Design review of the part built by this model. Coordinates are the model's own, in mm. Give positions to 0.01 mm unless a question says otherwise; leave off trailing zeros. Order: outer loops, then holes, each group sorted by start corner. A loop starts at its lowest first (then second) coordinate and runs counter-clockwise, first axis right, second up. Notation, with made-up numbers: M 0,62 L 42,62 A14 cw 42,79 Z; hole C 83,52.5 d7. An arc over 180 degrees is marked long. Put each result on its own line as item: value. Start each with the question number.
from build123d import *

# Parameters (mm, degrees)
BOSS_EXTRUDE1_DEPTH = 3.175
SKETCH4_R           = 2.1
SKETCH4_R_2         = 2.249999999
SKETCH4_R_3         = 2.25
CUT_EXTRUDE2_DEPTH  = 343.045224939


with BuildPart() as part:
    # Sketch2 → Boss-Extrude1 (new body)
    with BuildSketch(Plane.XY):
        with BuildLine():
            Line((-166.376823509, -157.21600002), (-166.376823509, -168.26500002))
            Line((-166.376823509, -168.26500002), (-167.519823509, -168.26500002))
            Line((-167.519823509, -168.26500002), (-167.519823509, -174.61500002))
            Line((-167.519823509, -174.61500002), (-163.058823509, -174.61500002))
            Line((-163.058823509, -174.61500002), (-163.058823509, -187.31500002))
            Line((-163.058823509, -187.31500002), (-167.519823509, -187.31500002))
            Line((-167.519823509, -187.31500002), (-167.519823509, -193.66500002))
            Line((-167.519823509, -193.66500002), (-166.376823509, -193.66500002))
            Line((-166.376823509, -193.66500002), (-166.376823509, -194.18100002))
            Line((-166.376823509, -194.18100002), (-148.199823509, -194.18100002))
            Line((-148.199823509, -194.18100002), (-148.199823509, -203.71400002))
            Line((-148.199823509, -203.71400002), (255.426176451, -203.71400002))
            Line((255.426176451, -203.71400002), (255.426176451, -194.18100002))
            Line((255.426176451, -194.18100002), (273.603176451, -194.18100002))
            Line((273.603176451, -194.18100002), (273.603176451, -193.66500002))
            Line((273.603176451, -193.66500002), (274.746176451, -193.66500002))
            Line((274.746176451, -193.66500002), (274.746176451, -187.31500002))
            Line((274.746176451, -187.31500002), (270.285176451, -187.31500002))
            Line((270.285176451, -187.31500002), (270.285176451, -174.61500002))
            Line((270.285176451, -174.61500002), (274.746176451, -174.61500002))
            Line((274.746176451, -174.61500002), (274.746176451, -168.26500002))
            Line((274.746176451, -168.26500002), (273.603176451, -168.26500002))
            Line((273.603176451, -168.26500002), (273.603176451, -157.21600002))
            Line((273.603176451, -157.21600002), (255.463301471, -157.21600002))
            Line((255.463301471, -157.21600002), (255.463301471, -160.70800002))
            ThreePointArc((255.463301471, -160.70800002), (254.533365501, -162.95306405), (252.288301471, -163.88300002))
            Line((252.288301471, -163.88300002), (242.288301471, -163.88300002))
            ThreePointArc((242.288301471, -163.88300002), (240.04323744, -162.95306405), (239.113301471, -160.70800002))
            Line((239.113301471, -160.70800002), (239.113301471, -157.21600002))
            Line((239.113301471, -157.21600002), (220.538301471, -157.21600002))
            Line((220.538301471, -157.21600002), (220.538301471, -160.70800002))
            ThreePointArc((220.538301471, -160.70800002), (219.608365501, -162.95306405), (217.363301471, -163.88300002))
            Line((217.363301471, -163.88300002), (207.363301471, -163.88300002))
            ThreePointArc((207.363301471, -163.88300002), (205.11823744, -162.95306405), (204.188301471, -160.70800002))
            Line((204.188301471, -160.70800002), (204.188301471, -157.21600002))
            Line((204.188301471, -157.21600002), (175.452051471, -157.21600002))
            Line((175.452051471, -157.21600002), (175.452051471, -160.70800002))
            ThreePointArc((175.452051471, -160.70800002), (174.522115501, -162.95306405), (172.277051471, -163.88300002))
            Line((172.277051471, -163.88300002), (162.277051471, -163.88300002))
            ThreePointArc((162.277051471, -163.88300002), (160.03198744, -162.95306405), (159.102051471, -160.70800002))
            Line((159.102051471, -160.70800002), (159.102051471, -157.21600002))
            Line((159.102051471, -157.21600002), (140.527051471, -157.21600002))
            Line((140.527051471, -157.21600002), (140.527051471, -160.70800002))
            ThreePointArc((140.527051471, -160.70800002), (139.597115501, -162.95306405), (137.352051471, -163.88300002))
            Line((137.352051471, -163.88300002), (127.352051471, -163.88300002))
            ThreePointArc((127.352051471, -163.88300002), (125.10698744, -162.95306405), (124.177051471, -160.70800002))
            Line((124.177051471, -160.70800002), (124.177051471, -157.21600002))
            Line((124.177051471, -157.21600002), (73.849301471, -157.21600002))
            Line((73.849301471, -157.21600002), (73.849301471, -160.70800002))
            ThreePointArc((73.849301471, -160.70800002), (72.919365501, -162.95306405), (70.674301471, -163.88300002))
            Line((70.674301471, -163.88300002), (60.674301471, -163.88300002))
            ThreePointArc((60.674301471, -163.88300002), (58.42923744, -162.95306405), (57.499301471, -160.70800002))
            Line((57.499301471, -160.70800002), (57.499301471, -157.21600002))
            Line((57.499301471, -157.21600002), (38.924301471, -157.21600002))
            Line((38.924301471, -157.21600002), (38.924301471, -160.70800002))
            ThreePointArc((38.924301471, -160.70800002), (37.994365501, -162.95306405), (35.749301471, -163.88300002))
            Line((35.749301471, -163.88300002), (25.749301471, -163.88300002))
            ThreePointArc((25.749301471, -163.88300002), (23.50423744, -162.95306405), (22.574301471, -160.70800002))
            Line((22.574301471, -160.70800002), (22.574301471, -157.21600002))
            Line((22.574301471, -157.21600002), (-6.161948529, -157.21600002))
            Line((-6.161948529, -157.21600002), (-6.161948529, -160.70800002))
            ThreePointArc((-6.161948529, -160.70800002), (-7.091884499, -162.95306405), (-9.336948529, -163.88300002))
            Line((-9.336948529, -163.88300002), (-19.336948529, -163.88300002))
            ThreePointArc((-19.336948529, -163.88300002), (-21.58201256, -162.95306405), (-22.511948529, -160.70800002))
            Line((-22.511948529, -160.70800002), (-22.511948529, -157.21600002))
            Line((-22.511948529, -157.21600002), (-41.086948529, -157.21600002))
            Line((-41.086948529, -157.21600002), (-41.086948529, -160.70800002))
            ThreePointArc((-41.086948529, -160.70800002), (-42.016884499, -162.95306405), (-44.261948529, -163.88300002))
            Line((-44.261948529, -163.88300002), (-54.261948529, -163.88300002))
            ThreePointArc((-54.261948529, -163.88300002), (-56.50701256, -162.95306405), (-57.436948529, -160.70800002))
            Line((-57.436948529, -160.70800002), (-57.436948529, -157.21600002))
            Line((-57.436948529, -157.21600002), (-107.764698529, -157.21600002))
            Line((-107.764698529, -157.21600002), (-107.764698529, -160.70800002))
            ThreePointArc((-107.764698529, -160.70800002), (-108.694634499, -162.95306405), (-110.939698529, -163.88300002))
            Line((-110.939698529, -163.88300002), (-120.939698529, -163.88300002))
            ThreePointArc((-120.939698529, -163.88300002), (-123.18476256, -162.95306405), (-124.114698529, -160.70800002))
            Line((-124.114698529, -160.70800002), (-124.114698529, -157.21600002))
            Line((-124.114698529, -157.21600002), (-142.689698529, -157.21600002))
            Line((-142.689698529, -157.21600002), (-142.689698529, -160.70800002))
            ThreePointArc((-142.689698529, -160.70800002), (-143.619634499, -162.95306405), (-145.864698529, -163.88300002))
            Line((-145.864698529, -163.88300002), (-155.864698529, -163.88300002))
            ThreePointArc((-155.864698529, -163.88300002), (-158.10976256, -162.95306405), (-159.039698529, -160.70800002))
            Line((-159.039698529, -160.70800002), (-159.039698529, -157.21600002))
            Line((-159.039698529, -157.21600002), (-166.376823509, -157.21600002))
        make_face()
    extrude(amount=BOSS_EXTRUDE1_DEPTH)

    # Sketch4 → Cut-Extrude2 (cut, through all)
    with BuildSketch(Plane.XY.offset(3.175)):
        with Locations((220.106176451, -182.10474)):
            Circle(SKETCH4_R)
        with Locations((173.906176451, -182.10474)):
            Circle(SKETCH4_R)
        with Locations((139.818076453, -197.329197783)):
            Circle(SKETCH4_R_2)
        with Locations((16.818076453, -197.329197783)):
            Circle(SKETCH4_R_2)
        with Locations((-4.519823509, -183.71400002)):
            Circle(SKETCH4_R_3)
        with Locations((-63.519823509, -183.71400002)):
            Circle(SKETCH4_R_3)
        with Locations((-103.723323529, -182.10474)):
            Circle(SKETCH4_R)
        with Locations((-149.923323529, -182.10474)):
            Circle(SKETCH4_R)
    extrude(amount=-CUT_EXTRUDE2_DEPTH, mode=Mode.SUBTRACT)


solid = part.part
1. Insertion check: pin 1 (1 mm diameter, centred on y = -162.5, z = 1.5, fed in from -X); pin 2 (1.6 mm diameter, centred on x = 267.5, z = 1, fed in from -Y); pin 3 (1 mm diameter, centred on x = -14.5, z = 2, fed in from +Y). Each pin has a flat end and moves straight along its axis. Give the tip position at first contact, or say it passes through.
2. Consider section B-B on z = 0.5. Give the number of separate pieces and of enclosed holes in the cut face, then the cut area to 3 significant figures.
3. Consider section A-A on x = 246.5. Give the boundary of the cut face in (y, z) (3 decimals).
4. To check wall thickness, follow probe 1 along X at (y, z) = (-197, 2.45); probe 2 along X at (y, z) = (-199, 1.3); probe 3 along X at (y, z) = (-180.5, 3). State the ranges of each line that lie inside material, in increasing order.
Returned:
1. pin 1: stops at x = -166.38
1. pin 2: stops at y = -194.18
1. pin 3: stops at y = -163.88
2. separate pieces: 1
2. enclosed holes: 8
2. area: 18,900 mm2
3. outline: M -203.714,0 L -163.883,0 L -163.883,3.175 L -203.714,3.175 Z
4. probe 1: x = -148.2 to 14.59, 19.04 to 137.59, 142.04 to 255.43
4. probe 2: x = -148.2 to 15.31, 18.33 to 138.31, 141.33 to 255.43
4. probe 3: x = -163.06 to -151.28, -148.57 to -105.08, -102.37 to 172.55, 175.26 to 218.75, 221.46 to 270.29
